Geometry: final body of the model. Coordinates: model frame, mm. A direction names the side the tool comes from. Give positions to 0.01 mm unless a question says otherwise; leave off trailing zeros. Write each loop counter-clockwise with the first axis right and the second up, starting at its lowest first coordinate (ties: lowest second). Pieces come first, ordered by that corner, then holes. Notation, with made-up numbers: M 54.25,-1.5 L 85.25,-1.5 A11 cw 85.25,7.5 Z; hole C -25,70.5 d11. An arc over 180 degrees is marked long. One line per question, with ' | ' between items.
from build123d import *

# Parameters (mm, degrees)
CYLINDER_R        = 4
CYLINDER_DEPTH    = 4.1
CYLINDER001_R     = 3.4
CYLINDER001_DEPTH = 1.2
BOX001_W          = 35.3
BOX001_H          = 15
BOX001_DEPTH      = 1
BOX_W             = 15
BOX_H             = 15
BOX_DEPTH         = 5.3


with BuildPart() as obj1:
    # Cylinder → Cylinder (new body)
    with BuildSketch(Plane.XY):
        Circle(CYLINDER_R)
    extrude(amount=CYLINDER_DEPTH)


with BuildPart() as obj2:
    # Cylinder001 → Cylinder001 (new body)
    with BuildSketch(Plane.XY.offset(4.1)):
        Circle(CYLINDER001_R)
    extrude(amount=CYLINDER001_DEPTH)

    # Fusion: union obj1
    add(obj1.part)


with BuildPart() as correa:
    # Box001 → Box001 (new body)
    with BuildSketch(Plane(origin=(-17.65, -7.5, 0), x_dir=(1, 0, 0), z_dir=(0, 0, 1))):
        with Locations((17.65, 7.5)):
            Rectangle(BOX001_W, BOX001_H)
    extrude(amount=BOX001_DEPTH)


with BuildPart() as cut:
    # Box → Box (new body)
    with BuildSketch(Plane(origin=(-7.5, -7.5, 0), x_dir=(1, 0, 0), z_dir=(0, 0, 1))):
        with Locations((7.5, 7.5)):
            Rectangle(BOX_W, BOX_H)
    extrude(amount=BOX_DEPTH)

    # Fusion001: union correa
    add(correa.part)

    # Cut: cut obj2
    add(obj2.part, mode=Mode.SUBTRACT)


solid = cut.part
(1) Cut plane A-A, the plane x = 0. Return loops of the section in (y, z), then the cut area to 3 significant figures.
Working result:
outline: M -7.5,0 L -4,0 L -4,4.1 L -3.4,4.1 L -3.4,5.3 L -7.5,5.3 Z; M 3.4,4.1 L 4,4.1 L 4,0 L 7.5,0 L 7.5,5.3 L 3.4,5.3 Z | area: 38.5 mm^2
(2) Material intervals for L1, parallel to Y at x = 0, z = 4.9; L2, parallel to Y at x = 0, z = 3.3; L3, parallel to Z at x = 14, y = -1, sorted ascending. Write a range as [from, to].
Working result:
L1: y = [-7.5, -3.4], [3.4, 7.5] | L2: y = [-7.5, -4], [4, 7.5] | L3: z = [0, 1]
(3) Draft query along Y for faces 4 (the face through (0, 7.5, 2)), 5 (the face through (-2, -3, 4.1)), 6 (the face through (-13, 0, 1)). Return one class per face: released by +Y, released by -Y, zero draft, split by the parting line, or undercut.
Working result:
face 4: released by +Y | face 5: undercut | face 6: zero draft
(4) Set-up query: faces 1 (the face through (-7.5, 0, 3)), 2 (the face through (-0.867, -3.905, 2.021)), 3 (the face through (7.5, 0, 3)). Return all of +Z, -Z, +X, -X, +Y, -Y with unobstructed straight access to the full face (end or side cutting, diameter ignored); none if empty.
Working result:
face 1: +Z, -X, +Y, -Y | face 2: -Z | face 3: +Z, +X, +Y, -Y
(5) Cut plane B-B, the plane z = 1.35. Return loops of the section in (x, y), then the cut area to 3 significant figures.
Working result:
outline: M -7.5,-7.5 L 7.5,-7.5 L 7.5,7.5 L -7.5,7.5 Z; hole C 0,0 d8 | area: 175 mm^2
(6) Cut plane C-C, the plane y = -5.5. Return loops of the section in (x, z), then the cut area to 3 significant figures.
Working result:
outline: M -17.65,0 L 17.65,0 L 17.65,1 L 7.5,1 L 7.5,5.3 L -7.5,5.3 L -7.5,1 L -17.65,1 Z | area: 99.8 mm^2
(7) Cut plane D-D, the plane y = -2.25. Return loops of the section in (x, z).
Working result:
outline: M -17.65,0 L -3.31,0 L -3.31,4.1 L -2.55,4.1 L -2.55,5.3 L -7.5,5.3 L -7.5,1 L -17.65,1 Z; M 2.55,4.1 L 3.31,4.1 L 3.31,0 L 17.65,0 L 17.65,1 L 7.5,1 L 7.5,5.3 L 2.55,5.3 Z
(8) First-contact query: P1, Ø4, axis at x = 12, y = 2, coming from the +Z side; P2, Ø3, axis at y = -2, z = 3.5, coming from the -X side; P3, Ø3, axis at y = -2.5, z = 3, coming from the +X side. Flat tips, straight axial feed; report the tip coordinate or a pass-through.
Working result:
P1: stops at z = 1 | P2: stops at x = -7.5 | P3: stops at x = 7.5
